Part model, mm, in its own coordinate system. Round coordinates to 2 decimals unless told otherwise and drop trailing zeros. Order: outer loops, then holes, each group sorted by start corner. A loop starts at its lowest first (then second) coordinate and runs counter-clockwise, first axis right, second up. Notation, with made-up numbers: M 21,-15 L 71,-15 A18 ccw 71,7 Z; hole C 7,64 d6. An arc over 180 degrees is marked long. One line per question, with ' | ' between items.
from build123d import *

# Parameters (mm, degrees)
SKETCH1_W           = 370
SKETCH1_H           = 260
BOSS_EXTRUDE1_DEPTH = 5
SKETCH3_W           = 53
SKETCH3_H           = 50
CUT_EXTRUDE3_DEPTH  = 10


with BuildPart() as part:
    # Sketch1 → Boss-Extrude1 (new body)
    with BuildSketch(Plane(origin=(0, 0, 0), x_dir=(1, 0, 0), z_dir=(0, 1, 0))):
        Rectangle(SKETCH1_W, SKETCH1_H)
    extrude(amount=BOSS_EXTRUDE1_DEPTH)

    # Sketch3 → Cut-Extrude3 (cut)
    with BuildSketch(Plane.XZ):
        with Locations((-139, 86)):
            Rectangle(SKETCH3_W, SKETCH3_H)
        with Locations((-139, -86)):
            Rectangle(SKETCH3_W, SKETCH3_H)
        with Locations((139, 86)):
            Rectangle(SKETCH3_W, SKETCH3_H)
        with Locations((139, -86)):
            Rectangle(SKETCH3_W, SKETCH3_H)
    extrude(amount=-CUT_EXTRUDE3_DEPTH, mode=Mode.SUBTRACT)


solid = part.part
1) Saw through at C-C (y = 1.55). List the corners of the cut face in (x, z), plus the area to 3 significant figures.
The answers:
outline: M -185,-130 L 185,-130 L 185,130 L -185,130 Z; hole M -165.5,-111 L -112.5,-111 L -112.5,-61 L -165.5,-61 Z; hole M -165.5,61 L -112.5,61 L -112.5,111 L -165.5,111 Z; hole M 112.5,-111 L 165.5,-111 L 165.5,-61 L 112.5,-61 Z; hole M 112.5,61 L 165.5,61 L 165.5,111 L 112.5,111 Z | area: 85,600 mm²
2) Probe line 1 (Z direction, x = -160, y = 4.35); line 2 (X direction, y = 0.6, z = 108.5). List the from-to ranges inside material, lowest first. Write a range as [from, to].
The answers:
line 1: z = [-130, -111], [-61, 61], [111, 130] | line 2: x = [-185, -165.5], [-112.5, 112.5], [165.5, 185]
3) Saw through at B-B (z = 76.5). List the corners of the cut face in (x, y).
The answers:
outline: M -185,0 L -165.5,0 L -165.5,5 L -185,5 Z; M -112.5,0 L 112.5,0 L 112.5,5 L -112.5,5 Z; M 165.5,0 L 185,0 L 185,5 L 165.5,5 Z
4) Saw through at A-A (x = -123). List the corners of the cut face in (y, z).
The answers:
outline: M 0,-130 L 5,-130 L 5,-111 L 0,-111 Z; M 0,-61 L 5,-61 L 5,61 L 0,61 Z; M 0,111 L 5,111 L 5,130 L 0,130 Z
